from build123d import *

# Parameters (mm, degrees)
F0_R     = 3
F0_R_2   = 6.25
F1_DEPTH = 25


with BuildPart() as f1:
    # F0 (on Top) → F1 (new body)
    with BuildSketch(Plane.XY):
        with BuildLine():
            Line((37, -5), (-34.773622, 19.465225))
            ThreePointArc((-34.773622, 19.465225), (-46.092599, 15.874508), (-46, 4))
            Line((-46, 4), (-28, -20))
            Line((-28, -20), (37, -20))
            Line((37, -20), (37, -5))
        make_face()
        with Locations((-17, -10)):
            Circle(F0_R, mode=Mode.SUBTRACT)
        with Locations((5, -10)):
            Circle(F0_R, mode=Mode.SUBTRACT)
        with Locations((27, -10)):
            Circle(F0_R, mode=Mode.SUBTRACT)
        with Locations((-20, 8)):
            Circle(F0_R, mode=Mode.SUBTRACT)
        with Locations((-38, 10)):
            Circle(F0_R_2, mode=Mode.SUBTRACT)
    extrude(amount=F1_DEPTH)


solid = f1.part
Work out the finished part from the listing and answer in its coordinate system (mm). Coordinates: 2 decimals unless noted, no trailing zeros. Write each loop counter-clockwise with the first axis right and the second up, starting at its lowest first coordinate (ties: lowest second). Pieces come first, ordered by that corner, then holes.
1. The part is cut by section D-D, the plane y = 8. Write down the section's boundary in (x, z), and give its area (3 significant figures).
Results list:
outline: (-47.8, 0) - (-43.92, 0) - (-43.92, 25) - (-47.8, 25) - close; (-32.08, 0) - (-23, 0) - (-23, 25) - (-32.08, 25) - close; (-17, 0) - (-1.14, 0) - (-1.14, 25) - (-17, 25) - close
area: 720 mm2
2. The part is cut by section B-B, the plane x = -38. Write down the section's boundary in (y, z), and give its area (3 significant figures).
Results list:
outline: (-6.67, 0) - (3.75, 0) - (3.75, 25) - (-6.67, 25) - close; (16.25, 0) - (20, 0) - (20, 25) - (16.25, 25) - close
area: 354 mm2
3. The part is cut by section A-A, the plane z = 20.5. Write down the section's boundary in (x, y).
Results list:
outline: (-46, 4) - (-28, -20) - (37, -20) - (37, -5) - (-34.77, 19.47) arc R10 ccw to start; hole circle Ø12.5 at (-38, 10); hole circle Ø6 at (-20, 8); hole circle Ø6 at (-17, -10); hole circle Ø6 at (5, -10); hole circle Ø6 at (27, -10)
4. For a pull along Y with two mould halves and no side action, classify faces 1 (the cylindrical face through (24, -10, 12)), 2 (the flat face through (-6, -4, 25)), 3 (the flat face through (1.62, 7.06, 12.32)), 4 (the flat face through (4, -20, 12)) as +Y half, -Y half, draft (parallel to the pull), parting line (faces both ways), or undercut.
Results list:
face 1: undercut
face 2: draft
face 3: +Y half
face 4: -Y half
5. Consider line 1 along Y through (x, z) = (-14.5, 16.5); line 2 along Y through (x, z) = (5, 15.75); line 3 along X through (y, z) = (-14.5, 9.25) (3 decimals). Determine where each line is inside the solid, lowest interval first.
Results list:
line 1: y = -20 to -11.66, -8.34 to 12.55
line 2: y = -20 to -13, -7 to 5.91
line 3: x = -32.125 to 37
6. The part is cut by section C-C, the plane y = -10. Write down the section's boundary in (x, z).
Results list:
outline: (-35.5, 0) - (-20, 0) - (-20, 25) - (-35.5, 25) - close; (-14, 0) - (2, 0) - (2, 25) - (-14, 25) - close; (8, 0) - (24, 0) - (24, 25) - (8, 25) - close; (30, 0) - (37, 0) - (37, 25) - (30, 25) - close
7. Flat-ended cylindrical pins translate along their axes: pin 1 (1 mm diameter, centred on y = 16, z = 4.5, fed in from -X); pin 2 (12 mm diameter, centred on y = -10, z = 9, fed in from -X); pin 3 (6 mm diameter, centred on x = -13, z = 20.5, fed in from +Y). Find the tip coordinate at first contact, or state that the pin passes through.
Results list:
pin 1: stops at x = -46.35
pin 2: stops at x = -40
pin 3: stops at y = 13.07
